Verification items for this drawing (mm, ordinates from the low corner). Round coordinates to 2 decimals unless told otherwise and drop trailing zeros. Order: outer loops, then holes, each group sorted by start corner. A loop starts at its lowest first (then second) coordinate and runs counter-clockwise, first axis right, second up. Notation, with made-up numbers: (-4, -8) -> (51, -8) arc R31 ccw to (51, 28) -> close; hole circle Ø9 at (-25.75, 31.25). An arc over 180 degrees is marked (long way). Answer in a Markdown table with one row per item. Add a question column.
1. Sectioned sample at B-B, the plane x = 9.75. Record the boundary of the cut face in (y, z).
2. Depth check by flat-ended pin: P1, Ø0.9, axis at x = 6, y = 1.5, coming from the -Z side; P2, Ø0.9, axis at x = 11.5, y = 3, coming from the +Z side. Enter the tip coordinate at first touch or a pass-through.
3. Material ranges on L1, parallel to Z at x = 6.75, y = 3.5; L2, parallel to X at y = 0.8, z = 54.5; L3, parallel to Z at x = 10, y = 4.65, recorded low to high. Write a range as from..to.
4. Sectioned sample at A-A, the plane z = 56. Record the boundary of the cut face in (x, y), then the cut area to 3 significant figures.
5. Sectioned sample at C-C, the plane y = 2.5. Count the separate pieces of the cut face and the enclosed holes in it, then the cut area to 3 significant figures.
6. Sectioned sample at D-D, the plane z = 9. Record the boundary of the cut face in (x, y).
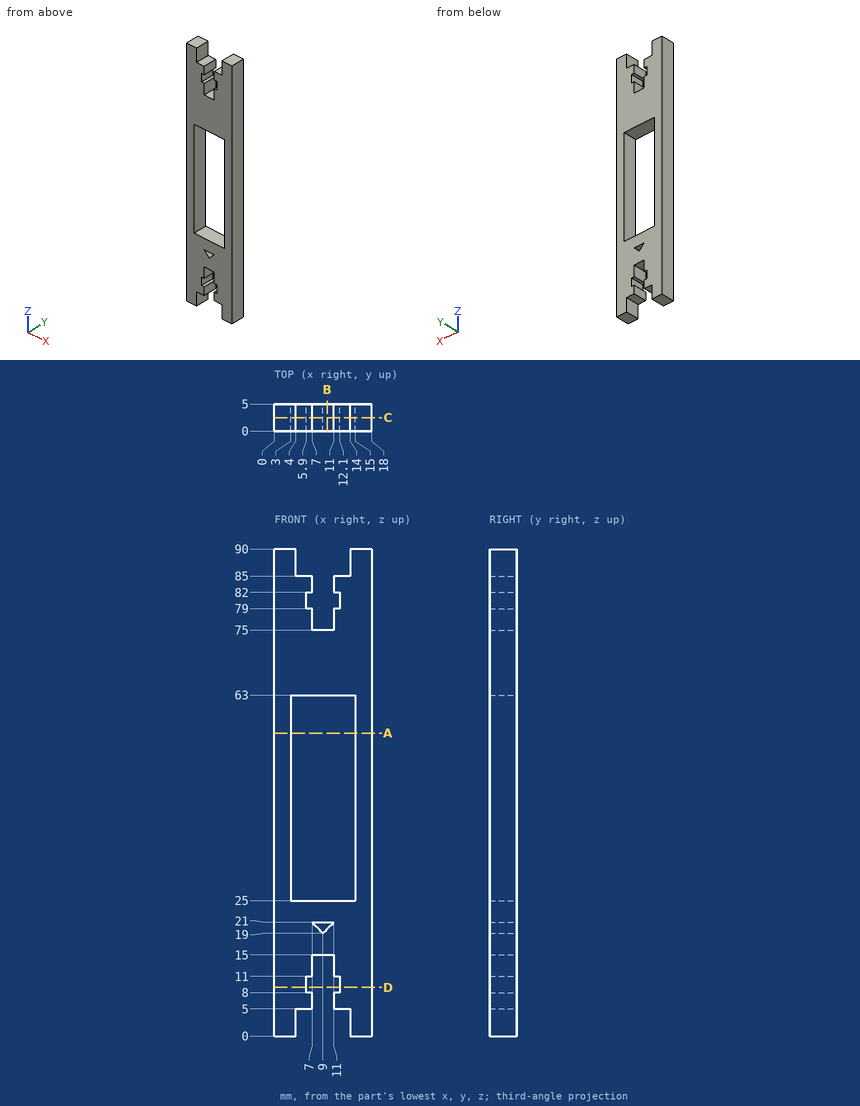
Answer key:
| question | item | result |
|---|---|---|
| 1 | outline | (0, 15) -> (5, 15) -> (5, 19.75) -> (0, 19.75) -> close; (0, 21) -> (5, 21) -> (5, 25) -> (0, 25) -> close; (0, 63) -> (5, 63) -> (5, 75) -> (0, 75) -> close |
| 2 | P1 | stops at z = 5 |
| 2 | P2 | stops at z = 85 |
| 3 | L1 | z = 5..8, 11..25, 63..79, 82..85 |
| 3 | L2 | x = 0..3, 15..18 |
| 3 | L3 | z = 15..20, 21..25, 63..75 |
| 4 | outline | (0, 0) -> (3, 0) -> (3, 5) -> (0, 5) -> close; (15, 0) -> (18, 0) -> (18, 5) -> (15, 5) -> close |
| 4 | area | 30.0 mm² |
| 5 | separate pieces | 1 |
| 5 | enclosed holes | 2 |
| 5 | area | 967 mm² |
| 6 | outline | (0, 0) -> (5.9, 0) -> (5.9, 5) -> (0, 5) -> close; (12.1, 0) -> (18, 0) -> (18, 5) -> (12.1, 5) -> close |
